Check sheet for the modelled part. Datum: model origin and axes. Units: mm. Face numbers are marked on the shaded views. Coordinates: 2 decimals unless noted, no trailing zeros. Loops run counter-clockwise (first coordinate to the right, second up) from the corner with the lowest first, then second, coordinate; pieces in that order, holes last.
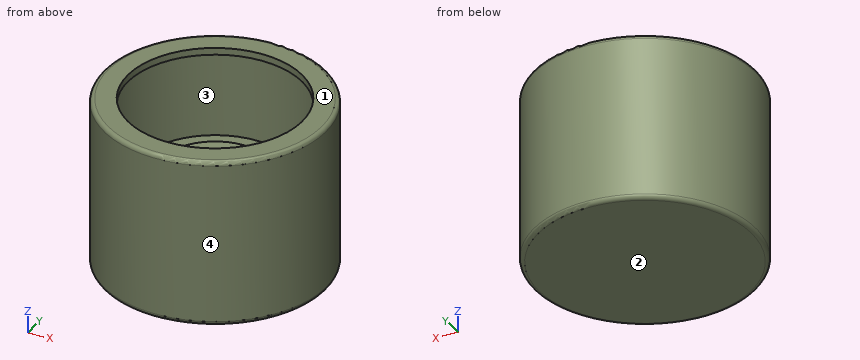
from build123d import *

# Parameters (mm, degrees)
SKETCH1_R           = 7.95
BOSS_EXTRUDE1_DEPTH = 12.1
FILLET1_R           = 0.3
SKETCH3_R           = 7.5
CUT_EXTRUDE2_DEPTH  = 10
SKETCH2_R           = 7.65
SKETCH2_R_2         = 6.25
BOSS_EXTRUDE2_DEPTH = 0.5
SKETCH4_R           = 5.5
BOSS_EXTRUDE3_DEPTH = 4


with BuildPart() as part:
    # Sketch1 → Boss-Extrude1 (new body)
    with BuildSketch(Plane.XY):
        Circle(SKETCH1_R)
    extrude(amount=BOSS_EXTRUDE1_DEPTH)

    # Fillet1
    fillet1_edges = [part.edges().sort_by_distance(p)[0] for p in [
        (-7.95, 0, 0),
        (-7.95, 0, 12.1),
    ]]
    fillet(fillet1_edges, radius=FILLET1_R)

    # Sketch3 → Cut-Extrude2 (cut)
    with BuildSketch(Plane.XY.offset(12.1)):
        Circle(SKETCH3_R)
    extrude(amount=-CUT_EXTRUDE2_DEPTH, mode=Mode.SUBTRACT)

    # Sketch2 → Boss-Extrude2 (add)
    with BuildSketch(Plane.XY.offset(12.1)):
        Circle(SKETCH2_R)
        Circle(SKETCH2_R_2, mode=Mode.SUBTRACT)
    extrude(amount=-BOSS_EXTRUDE2_DEPTH)

    # Sketch4 → Boss-Extrude3 (add)
    with BuildSketch(Plane.XY.offset(2.1)):
        Circle(SKETCH4_R)
    extrude(amount=BOSS_EXTRUDE3_DEPTH)

    # Sketch6 → Revolve2 (revolve)
    with BuildSketch(Plane(origin=(0, 0, 0), x_dir=(0, 0, -1), z_dir=(1, 0, 0))):
        with BuildLine():
            Line((-5.5, 3.790901005), (-5.5, 0))
            Line((-5.5, 0), (-6, 0))
            Line((-6, 0), (-6, 0.25))
            Line((-6, 0.25), (-6.119453289, 0.451240685))
            ThreePointArc((-6.119453289, 0.451240685), (-6.249755753, 0.734093475), (-6.318842572, 1.03775685))
            Line((-6.318842572, 1.03775685), (-6.65, 3.790901005))
            Line((-6.65, 3.790901005), (-5.5, 3.790901005))
        make_face()
    revolve(axis=Axis((0, 0, 0), (0, 0, 1)))


solid = part.part
(1) Gauge pin test, flat ends, axial feed: P1, Ø2, axis at x = -5, z = 6.5, coming from the -Y side; P2, Ø4, axis at x = -3.5, y = -6, coming from the -Z side; P3, Ø5.5, axis at x = 2, y = 0, coming from the +Z side; P4, Ø1.5, axis at y = 2.5, z = 9.5, coming from the -X side (3 decimals). Record the tip position at first contact, or that the pin passes through.
(2) Draft check along Z on the marked faces 1, 2, 3 and 4. Enter one of: pulls with the +Z half, pulls with the -Z half, needs draft (parallel to the pull), parting line crosses it, or undercut.
(3) Scan lines: line 1 along Y through (x, z) = (0, 4.5); line 2 along Y through (x, z) = (0, 9.5); line 3 along X through (y, z) = (2, 4.5). Record each from-to range of solid material in increasing order.
(4) Section check A-A, the plane z = 2.5. Enter the section's corners in (x, y), plus the area to 3 significant figures.
(5) Section check B-B, the plane z = 10. Enter the section's corners in (x, y).
Determined:
1. P1: stops at y = -6.87
1. P2: stops at z = 0
1. P3: stops at z = 6.65
1. P4: stops at x = -7.755
2. face 1: pulls with the +Z half
2. face 2: pulls with the -Z half
2. face 3: undercut
2. face 4: needs draft
3. line 1: y = -7.95 to -7.5, -5.5 to 5.5, 7.5 to 7.95
3. line 2: y = -7.95 to -7.5, 7.5 to 7.95
3. line 3: x = -7.69 to -7.23, -5.12 to 5.12, 7.23 to 7.69
4. outline: circle Ø15.9 at (0, 0); circle Ø11 at (0, 0); hole circle Ø15 at (0, 0)
4. area: 117 mm2
5. outline: circle Ø15.9 at (0, 0); hole circle Ø15 at (0, 0)
